Can you work these out from the model? Positions are in its coordinate system, mm. A direction names the side the tool comes from. Give positions to 0.01 mm unless a question says otherwise; leave off trailing zeros. Loops run counter-clockwise (first coordinate to the right, second up) from the corner with the lowest first, then second, coordinate; pieces in that order, holes last. Notation, with made-up numbers: (-39.5, 22.5) - (-29.5, 22.5) arc R23 cw to (-29.5, 60.5) - close; hole circle Ø11 at (0, 2). An arc over 180 degrees is marked (long way). Answer as a JSON object with one key per item and string values.
```python
from build123d import *

# Parameters (mm, degrees)
F1_DEPTH  = 1828.8
F3_DEPTH  = 19.05
F5_DEPTH  = 76.2
F7_DEPTH  = 57.15
F9_DEPTH  = 25.4
F12_DEPTH = 19.05


with BuildPart() as f1:
    # F0 (on Top) → F1 (new body)
    with BuildSketch(Plane.XY):
        Polygon((279.4, 279.4), (-279.4, 279.4), (-279.4, -279.4), (25.4, -279.4), (25.4, -260.35), (-260.35, -260.35), (-260.35, 260.35), (260.35, 260.35), (260.35, -25.4), (279.4, -25.4), align=None)
    extrude(amount=F1_DEPTH)

    # F2 (on face) → F3 (join)
    with BuildSketch(Plane.XY.offset(1828.8)):
        Polygon((-279.4, -279.4), (25.4, -279.4), (279.4, -25.4), (279.4, 279.4), (-279.4, 279.4), align=None)
    extrude(amount=-F3_DEPTH)

    # F4 (on Top) → F5 (join)
    with BuildSketch(Plane.XY):
        Polygon((-279.4, -279.4), (25.4, -279.4), (279.4, -25.4), (279.4, 279.4), (-279.4, 279.4), align=None)
    extrude(amount=F5_DEPTH)

    # F6 (on face) → F7 (cut)
    with BuildSketch(Plane(origin=(0, 0, 0), x_dir=(1, 0, 0), z_dir=(0, 0, -1))):
        Polygon((-260.35, -260.35), (260.35, -260.35), (260.35, 17.5092316368), (17.5092316368, 260.35), (-260.35, 260.35), align=None)
    extrude(amount=-F7_DEPTH, mode=Mode.SUBTRACT)

    # F8 (on face) → F9 (cut)
    with BuildSketch(Plane(origin=(152.4, -152.4, 0), x_dir=(0.7071067812, 0.7071067812, 0), z_dir=(0.7071067812, -0.7071067812, 0))):
        with BuildLine():
            Line((-127, 0), (127, 0))
            ThreePointArc((127, 0), (0, 34.0295474388), (-127, 0))
        make_face()
    extrude(amount=-F9_DEPTH, mode=Mode.SUBTRACT)

    # F11 (on offset) → F12 (join)
    with BuildSketch(Plane(origin=(0, 0, 914.4), x_dir=(1, 0, 0), z_dir=(0, 0, -1))):
        Polygon((-260.35, 260.35), (-260.35, -260.35), (260.35, -260.35), (260.35, 25.4), (25.4, 260.35), align=None)
    extrude(amount=F12_DEPTH)


solid = f1.part
```
1) If we mould it in two halves opening along Y, with no side actions, what happens to faces 4 (the flat face through (260.35, 123, 28)), 5 (the flat face through (-129, -279.4, 902)), 6 (the flat face through (-63, 270, 0))? For each: released by +Y, released by -Y, zero draft, split by the parting line, or undercut.
Check sheet entries:
{"face 4": "undercut", "face 5": "released by -Y", "face 6": "zero draft"}
2) I'm going to push flat-ended pins straight in: P1, Ø21, axis at x = 270, z = 1125, coming from the -Y side; P2, Ø5.5, axis at y = -266.5, z = 553, coming from the +X side; P3, Ø2, axis at y = -123, z = 1641, coming from the +X side. Where does each tip first touch, or does it pass through?
Check sheet entries:
{"P1": "y = -25.4", "P2": "x = 25.4", "P3": "x = -260.35"}
3) I need wall thicknesses on L1, parallel to Z at x = 154, y = 240.5; L2, parallel to X at y = 17, z = 476. Which ranges of each line are inside material? Lowest first, please.
Check sheet entries:
{"L1": "57.15 to 76.2, 895.35 to 914.4, 1809.75 to 1828.8", "L2": "-279.4 to -260.35, 260.35 to 279.4"}
4) Imagine slicing it at C-C on z = 1705. Write out the boundary of the cut face in (x, y).
Check sheet entries:
{"outline": "(-279.4, -279.4) - (25.4, -279.4) - (25.4, -260.35) - (-260.35, -260.35) - (-260.35, 260.35) - (260.35, 260.35) - (260.35, -25.4) - (279.4, -25.4) - (279.4, 279.4) - (-279.4, 279.4) - close"}
5) Which directions (+Z, -Z, +X, -X, +Y, -Y) give clear straight access to the entire face, cutting with the end or side of a thin tool? Please do faces 1 (the flat face through (260.35, 119, 1356)), 2 (the flat face through (-115, -260.35, 480)), 3 (the flat face through (144.52, -141.23, 905.01)).
Check sheet entries:
{"face 1": "-Y", "face 2": "+X", "face 3": "+X, -Y"}
6) Imagine slicing it at A-A on x = -39.5. Write out the boundary of the cut face in (y, z).
Check sheet entries:
{"outline": "(-279.4, 0) - (-260.35, 0) - (-260.35, 57.15) - (260.35, 57.15) - (260.35, 0) - (279.4, 0) - (279.4, 1828.8) - (-279.4, 1828.8) - close; hole (-260.35, 76.2) - (260.35, 76.2) - (260.35, 895.35) - (-260.35, 895.35) - close; hole (-260.35, 914.4) - (260.35, 914.4) - (260.35, 1809.75) - (-260.35, 1809.75) - close"}
